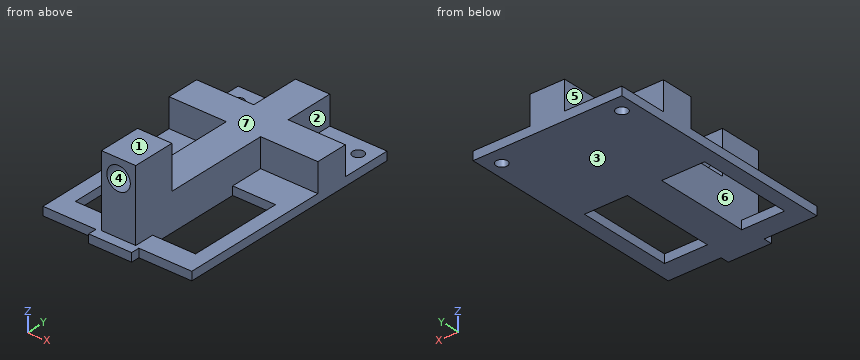
from build123d import *

# Parameters (mm, degrees)
F0_W     = 15
F0_H     = 33.2100428641
F0_W_2   = 15.0000001043
F0_R     = 2
F1_DEPTH = 3
F3_DEPTH = 10
F4_W     = 12
F4_H     = 15
F5_DEPTH = 15
F6_R     = 4.1
F7_DEPTH = 25


with BuildPart() as f1:
    # F0 (on Top) → F1 (new body)
    with BuildSketch(Plane.XY):
        Polygon((-36.0946140587, -40.7030668556), (-17.5946140587, -40.7030668556), (-17.5946140587, 40.2969331444), (-69.5946140587, 40.2969331444), (-69.5946140587, -40.7030668556), (-51.0946140587, -40.7030668556), align=None)
        with Locations((-57.0946140587, -16.605021432)):
            Rectangle(F0_W, F0_H, mode=Mode.SUBTRACT)
        with Locations((-30.0946140066, -16.605021432)):
            Rectangle(F0_W_2, F0_H, mode=Mode.SUBTRACT)
        with Locations((-64.5946140587, 34.2969331444)):
            Circle(F0_R, mode=Mode.SUBTRACT)
        with Locations((-22.5946139544, 34.2969331444)):
            Circle(F0_R, mode=Mode.SUBTRACT)
        Polygon((-36.0946140587, -43.7030668556), (-36.0946140587, -40.7030668556), (-51.0946140587, -40.7030668556), (-51.0946140587, -43.7030668556), (-43.5946140587, -43.7030668556), align=None)
    extrude(amount=F1_DEPTH)

    # F2 (on face) → F3 (join)
    with BuildSketch(Plane.XY.offset(3)):
        Polygon((-49.5946140587, 11.6144362837), (-49.5946140587, 0), (-49.5946140587, -33.2100428641), (-49.5946140587, -40.2100428641), (-37.5946140587, -40.2100428641), (-37.5946140587, -33.2100428641), (-37.5946140587, 0), (-37.5946140587, 11.6144362837), (-17.5946140587, 11.6144362837), (-17.5946140587, 23.017546162), (-37.5946140587, 23.017546162), (-37.5946140587, 40.2969331444), (-49.5946140587, 40.2969331444), (-49.5946140587, 23.017546162), (-69.5946140587, 23.017546162), (-69.5946140587, 11.6144362837), align=None)
    extrude(amount=F3_DEPTH)

    # F4 (on face) → F5 (join)
    with BuildSketch(Plane.XY.offset(13)):
        with Locations((-43.5946140587, -32.7100428641)):
            Rectangle(F4_W, F4_H)
    extrude(amount=F5_DEPTH)

    # F6 (on face) → F7 (cut)
    with BuildSketch(Plane(origin=(0, -25.2100428641, 0), x_dir=(-1, 0, 0), z_dir=(0, 1, 0))):
        with Locations((43.5946140587, 21.6)):
            Circle(F6_R)
    extrude(amount=-F7_DEPTH, mode=Mode.SUBTRACT)


solid = f1.part
Can you work these out from the model? Positions are in its coordinate system, mm. Face numbers are marked on the shaded views. A direction names the side the tool comes from. Coordinates: 2 decimals unless noted, no trailing zeros. Write each loop counter-clockwise with the first axis right and the second up, starting at its lowest first coordinate (ties: lowest second). Pieces come first, ordered by that corner, then holes. Notation, with made-up numbers: (57.25, 79.5) -> (63.25, 79.5) arc R26 ccw to (63.25, 118.5) -> close; hole circle Ø9 at (7.25, 77). An arc over 180 degrees is marked (long way). Answer as CSV lines item,"result".
1) On a 3-axis mill with a long thin cutter (end or side, diameter ignored), from which of +Z, -Z, +X, -X, +Y, -Y can I reach the whole of each face in a straight line? I mean the marked faces 5, 6 and 7. Say none if no direction works.
Check result:
face 5,"+Z, -X, +Y"
face 6,"+Z"
face 7,"+Z, +X, -X, +Y"
2) If we mould it in two halves opening along Z, with no side actions, what happens to the marked faces 1, 2, 3 and 4? For each: +Z half, -Z half, draft (parallel to the pull), parting line (faces both ways), or undercut.
Check result:
face 1,"+Z half"
face 2,"draft"
face 3,"-Z half"
face 4,"undercut"
3) Will these pins go through, and if not, where does the flat tip stop? P1, Ø1.5, axis at x = -55.5, z = 9.5, coming from the -Y side; P2, Ø5, axis at x = -41, z = 14, coming from the +Y side; P3, Ø1.5, axis at x = -57, z = 1.5, coming from the -Y side; P4, Ø6.5, axis at x = -64.59, y = 34.3, coming from the +Z side.
Check result:
P1,"y = 11.61"
P2,"y = 40.3"
P3,"y = -40.7"
P4,"z = 3"
4) If we section it at D-D on z = 7.25: Please give me the cut outline in (x, y).
Check result:
outline,"(-69.59, 11.61) -> (-49.59, 11.61) -> (-49.59, -40.21) -> (-37.59, -40.21) -> (-37.59, 11.61) -> (-17.59, 11.61) -> (-17.59, 23.02) -> (-37.59, 23.02) -> (-37.59, 40.3) -> (-49.59, 40.3) -> (-49.59, 23.02) -> (-69.59, 23.02) -> close"
5) If we section it at A-A on z = 21.6: Please give me the cut outline in (x, y), then the cut area to 3 significant figures.
Check result:
outline,"(-49.59, -40.21) -> (-47.69, -40.21) -> (-47.69, -25.21) -> (-49.59, -25.21) -> close; (-39.49, -40.21) -> (-37.59, -40.21) -> (-37.59, -25.21) -> (-39.49, -25.21) -> close"
area,"57.0 mm²"
6) If I drill on line 1 (Y direction, x = -41, z = 25.25); line 2 (Z direction, x = -44, y = -4); line 3 (Y direction, x = -53.5, z = 2), over which ranges is the centre line in solid material (lowest first)? Write a range as from..to.
Check result:
line 1,"-40.21..-25.21"
line 2,"0..13"
line 3,"-40.7..-33.21, 0..40.3"
7) If we section it at B-B on x = -34: Please give me the cut outline in (y, z), then the cut area to 3 significant figures.
Check result:
outline,"(-40.7, 0) -> (-33.21, 0) -> (-33.21, 3) -> (-40.7, 3) -> close; (0, 0) -> (40.3, 0) -> (40.3, 3) -> (23.02, 3) -> (23.02, 13) -> (11.61, 13) -> (11.61, 3) -> (0, 3) -> close"
area,"257 mm²"
8) If we section it at C-C on y = 1: Please give me the cut outline in (x, z), then the cut area to 3 significant figures.
Check result:
outline,"(-69.59, 0) -> (-17.59, 0) -> (-17.59, 3) -> (-37.59, 3) -> (-37.59, 13) -> (-49.59, 13) -> (-49.59, 3) -> (-69.59, 3) -> close"
area,"276 mm²"
